Build history of the part. All positions in model axes, mm. Face numbers are marked on the shaded views. A direction names the side the tool comes from. Give positions to 0.01 mm unless a question says otherwise; leave off trailing zeros. Loops run counter-clockwise (first coordinate to the right, second up) from the corner with the lowest first, then second, coordinate; pieces in that order, holes last. Notation, with made-up numbers: (-36.5, 54) -> (4.5, 54) arc R28 cw to (4.5, 73) -> close; hole circle Ø4 at (-40, 70.5). An arc over 180 degrees is marked (long way). Answer as a JSON object with one key per item and string values. Group by question number.
from build123d import *

# Parameters (mm, degrees)
F1_DEPTH = 27.5
F2_W     = 92
F2_H     = 160
F3_DEPTH = 26
F5_START = 20
F5_DEPTH = 7.5
F8_W     = 133
F8_H     = 6
F9_DEPTH = 27.5


# Not quite as in the source:
# - a feature names something its author has since deleted; it is built from what else it names


with BuildPart() as f1:
    # F0 (on Front) → F1 (new body, symmetric)
    with BuildSketch(Plane.XZ):
        with BuildLine():
            Line((-47.5, -75), (47.5, -75))
            Line((47.5, -75), (47.5, 75))
            Line((47.5, 75), (28.5, 75))
            add(Edge.make_bspline(
                [(0, -62.5), (28.5, -62.5), (28.5, 75)],
                knots=[0, 0, 0, 1.5707963268, 1.5707963268, 1.5707963268], degree=2, weights=[1, 0.7071067812, 1]))
            add(Edge.make_bspline(
                [(-28.5, 75), (-28.5, -62.5), (0, -62.5)],
                knots=[4.7123889804, 4.7123889804, 4.7123889804, 6.2831853072, 6.2831853072, 6.2831853072], degree=2, weights=[1, 0.7071067812, 1]))
            Line((-28.5, 75), (-47.5, 75))
            Line((-47.5, 75), (-47.5, -75))
        make_face()
    extrude(amount=F1_DEPTH, both=True)

    # F2 (on Front) → F3 (cut, symmetric)
    with BuildSketch(Plane.XZ):
        with Locations((0.2383571118, 6.4966206347)):
            Rectangle(F2_W, F2_H)
    extrude(amount=F3_DEPTH, both=True, mode=Mode.SUBTRACT)

    # F4 (on Front) → F5 (join)
    with BuildSketch(Plane.XZ.offset(F5_START)):
        with BuildLine():
            add(Edge.make_bspline(
                [(53.0086401116, 75), (53.7921645124, -12.5080782441), (49.3814773033, -67.453669192), (66.5, -69.7422416255)],
                knots=[0, 0, 0, 0, 145.3696436758, 145.3696436758, 145.3696436758, 145.3696436758], degree=3))
            Line((53.0086401116, 75), (47.5, 75))
            Line((47.5, 75), (47.5, -75))
            Line((47.5, -75), (66.5, -75))
            Line((66.5, -75), (66.5, -69.7422416255))
        make_face()
    extrude(amount=F5_DEPTH)

    # F6: F1 across plane


with BuildPart() as f1_1:
    add(f1.part)
    add(f1.part.mirror(Plane.YZ))

    # F7: F1 across plane


with BuildPart() as f1_2:
    add(f1_1.part)
    add(f1_1.part.mirror(Plane.XZ))

    # F8 (on Front) → F9 (join, symmetric)
    with BuildSketch(Plane.XZ):
        with Locations((0, -78)):
            Rectangle(F8_W, F8_H)
    extrude(amount=F9_DEPTH, both=True)


solid = f1_2.part
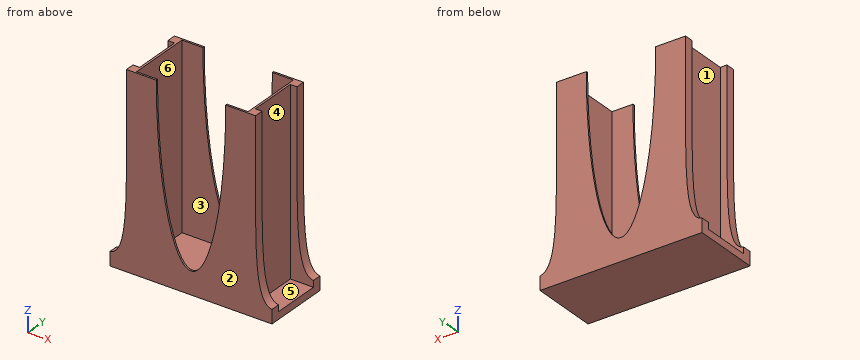
(1) Pull direction X, two halves, no side cores. Call the marked faces 4, 5 and 6: pulls with the +X half, pulls with the -X half, needs draft (parallel to the pull), parting line crosses it, or undercut.
(2) Saw through at C-C on x = 34. List the corners of the cut face in (y, z).
(3) Saw through at B-B on y = -16. List the corners of the cut face in (x, z), plus the area to 3 significant figures.
(4) 3-axis set-ups, long thin cutter, end or side, ignore diameter. For the marked faces 1, 2 and 3: which of +Z, -Z, +X, -X, +Y, -Y reach the whole face in a straight line?
(5) Probe line 1 along X through (y, z) = (17, -41.5); line 2 along Y through (x, z) = (-35, -26.5); line 3 along Z through (x, y) = (-19.5, -19.5). List the from-to ranges inside material, lowest first. Write a range as [from, to].
(6) Pin check, flat tips, straight feed: pin 1 (9.5 mm diameter, centred on x = 55.5, z = -20.5, fed in from +Y); pin 2 (15.5 mm diameter, centred on y = -8.5, z = -3, fed in from +X); pin 3 (6 mm diameter, centred on y = -0.5, z = 14, fed in from -X); pin 4 (5.5 mm diameter, centred on x = 52.5, y = -7, fed in from +Z). Stop position of each tip, or through.
(7) Saw through at A-A on x = 50.5. List the corners of the cut face in (y, z), plus the area to 3 significant figures.
Calculated:
{
 "1": {"face 4": "pulls with the +X half", "face 5": "needs draft", "face 6": "undercut"},
 "2": {"outline": "(-27.5, -81) -> (27.5, -81) -> (27.5, 75) -> (26, 75) -> (26, -73.5) -> (-26, -73.5) -> (-26, 75) -> (-27.5, 75) -> close"},
 "3": {"outline": "(-66.5, -81) -> (66.5, -81) -> (66.5, -75) -> (47.5, -75) -> (47.5, 75) -> (45.76, 75) -> (45.76, -73.5) -> (-45.76, -73.5) -> (-45.76, 75) -> (-47.5, 75) -> (-47.5, -75) -> (-66.5, -75) -> close", "area": "1,460 mm^2"},
 "4": {"face 1": "+Z, -X", "face 2": "+Z, -Z, +X, -X, -Y", "face 3": "+Z"},
 "5": {"line 1": "x = [-47.5, -45.76], [45.76, 47.5]", "line 2": "y = [-27.5, -26], [26, 27.5]", "line 3": "z = [-81, -73.5]"},
 "6": {"pin 1": "stops at y = 27.5", "pin 2": "stops at x = 47.5", "pin 3": "stops at x = -47.5", "pin 4": "stops at z = -75"},
 "7": {"outline": "(-27.5, -81) -> (27.5, -81) -> (27.5, 75) -> (20, 75) -> (20, -75) -> (-20, -75) -> (-20, 75) -> (-27.5, 75) -> close", "area": "2,580 mm^2"}
}
